Read the model definition and answer for the solid it produces. Units are mm, in the model's axes. Coordinates: 2 decimals unless noted, no trailing zeros. Order: outer loops, then holes, each group sorted by start corner. A loop starts at its lowest first (then second) coordinate and runs counter-clockwise, first axis right, second up. Notation, with made-up numbers: (19.25, 63) -> (67.25, 63) arc R10 cw to (67.25, 82) -> close; hole circle Ø4 at (24, -35). An arc over 180 degrees is marked (long way). Use CSV: the item, a comma, the result in double quotes.
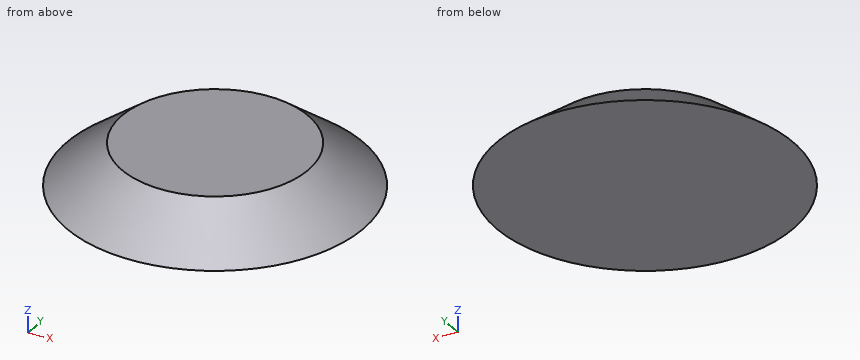
```python
from build123d import *

# Parameters (mm, degrees)
SKETCH_1_R      = 44
EXTRUDE_1_DEPTH = 20
SKETCH_4_R      = 70


with BuildPart() as part:
    # 草图1 → 凸台-拉伸1 (new body)
    with BuildSketch(Plane.XY):
        Circle(SKETCH_1_R)
    extrude(amount=EXTRUDE_1_DEPTH)

    # 草图4 → section 1 of loft_3
    with BuildSketch(Plane(origin=(0, 0, 0), x_dir=(-1, 0, 0), z_dir=(0, 0, -1)), mode=Mode.PRIVATE) as loft_3_s1:
        Circle(SKETCH_4_R)
    # loft up to a face of the part (loft_3)
    loft([Face(Wire([part.edges().sort_by_distance((-30.120072661, 32.074619607, 20))[0]])), loft_3_s1.sketch])


solid = part.part
```
Item 1: Straight lines are drawn through the part: line 1 along X through (y, z) = (12, 12.5); line 2 along Z through (x, y) = (48.5, 1); line 3 along X through (y, z) = (-18.5, 5). For each, find the intervals that lie inside material, in ascending order.
Return value:
line 1,"x = -52.39 to 52.39"
line 2,"z = 0 to 16.53"
line 3,"x = -60.75 to 60.75"
Item 2: Find section C-C, the plane z = 2. Give the vertices of the cut face in (x, y).
Return value:
outline,"circle Ø134.8 at (0, 0)"
Item 3: Each of these flat-tipped pins is pushed along its axis until it touches: P1, Ø4, axis at x = -46.5, z = 8.5, coming from the +Y side; P2, Ø2, axis at y = -45.5, z = 8, coming from the -X side; P3, Ø2, axis at x = -48, z = 8, coming from the +Y side. Where does it stop, or does it pass through?
Return value:
P1,"stops at y = 40.93"
P2,"stops at x = -40.78"
P3,"stops at y = 37.83"
Item 4: Find section A-A, the plane x = 0. Give the vertices of the cut face in (y, z), then the cut area to 3 significant figures.
Return value:
outline,"(-70, 0) -> (70, 0) -> (44, 20) -> (-44, 20) -> close"
area,"2,280 mm^2"
Item 5: Find section B-B, the plane z = 13.5. Give the vertices of the cut face in (x, y).
Return value:
outline,"circle Ø104.9 at (0, 0)"
